Input: part model. Units: mm. Frame: model coordinates. Give positions to 0.01 mm unless a question says otherwise; leave off trailing zeros. Order: outer loops, then holes, each group sorted by start corner. A loop starts at its lowest first (then second) coordinate and runs counter-clockwise, first axis right, second up. Notation, with made-up numbers: M 71,48 L 103,48 A19 cw 103,76 Z; hole C -10,33.25 d9. An arc over 180 degrees is marked long. Use a Markdown table: item, result.
from build123d import *

# Parameters (mm, degrees)
F0_R     = 9.95
F1_DEPTH = 3


with BuildPart() as f1:
    # F0 (on Top) → F1 (new body)
    with BuildSketch(Plane.XY):
        with BuildLine():
            ThreePointArc((7.292575, 13.10795), (0, 38.95), (-7.292575, 13.10795))
            ThreePointArc((-7.292575, 13.10795), (-10.52197, 10.690564), (-12.990381, 7.5))
            ThreePointArc((-12.990381, 7.5), (-14.519285, 3.767011), (-14.998105, -0.23842))
            ThreePointArc((-14.998105, -0.23842), (-33.731689, -19.475), (-7.70553, -12.86953))
            ThreePointArc((-7.70553, -12.86953), (-3.997315, -14.457575), (0, -15))
            ThreePointArc((0, -15), (3.997315, -14.457575), (7.70553, -12.86953))
            ThreePointArc((7.70553, -12.86953), (33.731689, -19.475), (14.998105, -0.23842))
            ThreePointArc((14.998105, -0.23842), (14.519285, 3.767011), (12.990381, 7.5))
            ThreePointArc((12.990381, 7.5), (10.52197, 10.690564), (7.292575, 13.10795))
        make_face()
        with Locations((-21.650635, -12.5)):
            Circle(F0_R, mode=Mode.SUBTRACT)
        with Locations((21.650635, -12.5)):
            Circle(F0_R, mode=Mode.SUBTRACT)
        with BuildLine():
            ThreePointArc((0, 11), (5.5, 9.526279), (9.526279, 5.5))
            ThreePointArc((9.526279, 5.5), (9.526279, -5.5), (0, -11))
            ThreePointArc((0, -11), (-9.526279, -5.5), (-9.526279, 5.5))
            ThreePointArc((-9.526279, 5.5), (-5.5, 9.526279), (0, 11))
        make_face(mode=Mode.SUBTRACT)
        with BuildLine():
            ThreePointArc((9.95, 25), (7.035712, 17.964288), (0, 15.05))
            ThreePointArc((0, 15.05), (-7.035712, 32.035712), (9.95, 25))
        make_face(mode=Mode.SUBTRACT)
    extrude(amount=F1_DEPTH)


solid = f1.part
1) Cut plane C-C on y = -6. Return loops of the section in (x, z).
Response values:
| item | result |
|---|---|
| outline | M -33.99,0 L -29.18,0 L -29.18,3 L -33.99,3 Z; M -14.12,0 L -9.22,0 L -9.22,3 L -14.12,3 Z; M 9.22,0 L 14.12,0 L 14.12,3 L 9.22,3 Z; M 29.18,0 L 33.99,0 L 33.99,3 L 29.18,3 Z |
2) Cut plane A-A on x = -21. Return loops of the section in (y, z), and give its area (3 significant figures).
Response values:
| item | result |
|---|---|
| outline | M -26.43,0 L -22.43,0 L -22.43,3 L -26.43,3 Z; M -2.57,0 L 1.43,0 L 1.43,3 L -2.57,3 Z |
| area | 24.0 mm² |
3) First-contact query: pin 1 Ø10 at (x, y) = (-26.5, -6.5) entering from -Z. Flat tip, straight axial feed; report the tip coordinate or a pass-through.
Response values:
| item | result |
|---|---|
| pin 1 | stops at z = 0 |
4) Cut plane D-D on x = 3. Return loops of the section in (y, z).
Response values:
| item | result |
|---|---|
| outline | M -14.7,0 L -10.58,0 L -10.58,3 L -14.7,3 Z; M 10.58,0 L 15.51,0 L 15.51,3 L 10.58,3 Z; M 34.49,0 L 38.62,0 L 38.62,3 L 34.49,3 Z |
5) Mould query, pull axis X, two halves, no side actions, for faces 1 (the face through (-11, -3, 3)), 2 (the face through (-33.98, -19.03, 1.48)), 3 (the face through (13.75, -18.55, 1.48)). Classes: released by +X, released by -X, zero draft, split by the parting line, or undercut.
Response values:
| item | result |
|---|---|
| face 1 | zero draft |
| face 2 | undercut |
| face 3 | undercut |
6) Material intervals for line 1 (X direction, y = -12, z = 2.85); line 2 (X direction, y = 25, z = 2.3); line 3 (X direction, y = -10, z = 1), sorted ascending. Write a range as from..to.
Response values:
| item | result |
|---|---|
| line 1 | x = -35.59..-31.59, -11.71..11.71, 31.59..35.59 |
| line 2 | x = -13.95..-9.95, 9.95..13.95 |
| line 3 | x = -35.37..-31.28, -12.02..-4.58, 4.58..12.02, 31.28..35.37 |
7) Cut plane B-B on z = 1.85. Return loops of the section in (x, y).
Response values:
| item | result |
|---|---|
| outline | M -15,-0.24 A13.95 ccw long -7.71,-12.87 A15 ccw 0,-15 A15 ccw 7.71,-12.87 A13.95 ccw long 15,-0.24 A15 ccw 12.99,7.5 A15 ccw 7.29,13.11 A13.95 ccw long -7.29,13.11 A15 ccw -12.99,7.5 A15 ccw Z; hole C -21.65,-12.5 d19.9; hole M -9.53,5.5 A11 ccw long 9.53,5.5 A11 ccw 0,11 A11 ccw Z; hole M 0,15.05 A9.95 ccw 9.95,25 A9.95 ccw long Z; hole C 21.65,-12.5 d19.9 |
